from build123d import *

# Parameters (mm, degrees)
SALIENTE_EXTRUIR1_DEPTH     = 180
REDONDEO1_R                 = 100
REDONDEO2_R                 = 10
CROQUIS2_W                  = 140
CROQUIS2_H                  = 70
CORTAR_EXTRUIR4_DEPTH       = 90
CROQUIS3_R                  = 30
CORTAR_EXTRUIR5_DEPTH       = 242.078733734
CORTAR_EXTRUIR6_DEPTH       = 282.806134391
CROQUIS5_W                  = 80.263157895
CROQUIS5_H                  = 10
CORTAR_EXTRUIR8_DEPTH       = 70
CROQUIS6_W                  = 80.263157895
CROQUIS6_H                  = 10
CORTAR_EXTRUIR9_DEPTH       = 243.676183384
REDONDEO8_R                 = 10
CORTAR_EXTRUIR10_DEPTH      = 242.078733734
CORTAR_EXTRUIR10_DEPTH_BACK = 242.078733734
CROQUIS8_W                  = 140
CROQUIS8_H                  = 70
SALIENTE_EXTRUIR2_DEPTH     = 10
CROQUIS9_R                  = 18.735611047
CORTAR_EXTRUIR11_DEPTH      = 282.806134525
REDONDEO9_R                 = 10


# Some blends are built 0.0001 mm under size
with BuildPart() as part:
    # Croquis1 → Saliente-Extruir1 (new body)
    with BuildSketch(Plane.XY):
        Polygon((-15.059146237, -60.657894737), (84.940853763, -60.657894737), (84.940853763, 29.342105263), (4.677695868, 29.342105263), (4.677695868, 139.342105263), (-15.059146237, 139.342105263), align=None)
    extrude(amount=SALIENTE_EXTRUIR1_DEPTH)

    # Redondeo1
    # the kernel refuses this fillet: 100 mm, written as the material it takes off along each edge
    with BuildSketch(Plane(origin=(254.677695868, 139.342105263, 180), x_dir=(0, 0, -1), z_dir=(-1, 0, 0))) as redondeo1_piece_1:
        with BuildLine():
            CenterArc((REDONDEO1_R, REDONDEO1_R), REDONDEO1_R, 180, 90)
            Line((0, REDONDEO1_R), (0, 0))
            Line((0, 0), (REDONDEO1_R, 0))
        make_face()
    extrude(amount=519.736842105, mode=Mode.SUBTRACT)
    with BuildSketch(Plane(origin=(254.677695868, 139.342105263, 0), x_dir=(0, 0, 1), z_dir=(-1, 0, 0))) as redondeo1_piece_2:
        with BuildLine():
            CenterArc((REDONDEO1_R, -REDONDEO1_R), REDONDEO1_R, 90, 90)
            Line((0, -REDONDEO1_R), (0, 0))
            Line((0, 0), (REDONDEO1_R, 0))
        make_face()
    extrude(amount=519.736842105, mode=Mode.SUBTRACT)

    # Redondeo2
    redondeo2_edges = [part.edges().sort_by_distance(p)[0] for p in [
        (44.809274816, 29.342105263, 180),
        (44.809274816, 29.342105263, 0),
    ]]
    fillet(redondeo2_edges, radius=REDONDEO2_R)

    # Croquis2 → Cortar-Extruir4 (cut)
    with BuildSketch(Plane(origin=(84.940853763, 0, 0), x_dir=(0, 0, -1), z_dir=(1, 0, 0))):
        with Locations((-90, -5.657894737)):
            Rectangle(CROQUIS2_W, CROQUIS2_H)
    extrude(amount=-CORTAR_EXTRUIR4_DEPTH, mode=Mode.SUBTRACT)

    # Croquis3 → Cortar-Extruir5 (cut, through all)
    with BuildSketch(Plane(origin=(4.677695868, 0, 0), x_dir=(0, 0, -1), z_dir=(1, 0, 0))):
        with Locations((-90, 93.548562432)):
            Circle(CROQUIS3_R)
    extrude(amount=-CORTAR_EXTRUIR5_DEPTH, mode=Mode.SUBTRACT)

    # Croquis4 → Cortar-Extruir6 (cut, through all)
    with BuildSketch(Plane(origin=(0, -60.657894737, 0), x_dir=(-1, 0, 0), z_dir=(0, -1, 0))):
        with BuildLine():
            Line((-58.010173511, -150), (-58.010173511, -120))
            ThreePointArc((-58.010173511, -120), (-38.975513637, -100.965340126), (-19.940853763, -120))
            Line((-19.940853763, -120), (-19.940853763, -150))
            ThreePointArc((-19.940853763, -150), (-38.975513637, -169.034659874), (-58.010173511, -150))
        make_face()
        with BuildLine():
            Line((-58.010173511, -60), (-58.010173511, -30))
            ThreePointArc((-58.010173511, -30), (-38.975513637, -10.965340126), (-19.940853763, -30))
            Line((-19.940853763, -30), (-19.940853763, -60))
            ThreePointArc((-19.940853763, -60), (-38.975513637, -79.034659874), (-58.010173511, -60))
        make_face()
    extrude(amount=-CORTAR_EXTRUIR6_DEPTH, mode=Mode.SUBTRACT)

    # Croquis5 → Cortar-Extruir8 (cut)
    with BuildSketch(Plane(origin=(0, 29.342105263, 0), x_dir=(1, 0, 0), z_dir=(0, 1, 0))):
        with Locations((44.809274816, -15)):
            Rectangle(CROQUIS5_W, CROQUIS5_H)
        with Locations((44.809274816, -165)):
            Rectangle(CROQUIS5_W, CROQUIS5_H)
    extrude(amount=-CORTAR_EXTRUIR8_DEPTH, mode=Mode.SUBTRACT)

    # Croquis6 → Cortar-Extruir9 (cut, through all)
    with BuildSketch(Plane.XY.offset(180)):
        with Locations((44.809274816, 24.342105263)):
            Rectangle(CROQUIS6_W, CROQUIS6_H)
    extrude(amount=-CORTAR_EXTRUIR9_DEPTH, mode=Mode.SUBTRACT)

    # Redondeo8
    redondeo8_edges = [part.edges().sort_by_distance(p)[0] for p in [
        (84.940853763, 19.342105263, 175),
        (84.940853763, 19.342105263, 5),
    ]]
    fillet(redondeo8_edges, radius=REDONDEO8_R)

    # Croquis7 → Cortar-Extruir10 (cut, two sides: drawn at the far end of the back side and taken through both)
    with BuildSketch(Plane(origin=(4.677695868, 0, 0), x_dir=(0, 0, -1), z_dir=(1, 0, 0)).offset(-CORTAR_EXTRUIR10_DEPTH_BACK)):
        with BuildLine():
            add(Edge.make_bspline(
                [(-113.081277055, 133.711746083), (-124.698414262, 126.957224262), (-152.328432442, 87.000878261), (-154.754506131, 42.525291557), (-180, 19.342105263)],
                knots=[0.150275034, 0.150275034, 0.150275034, 0.150275034, 0.412965146, 1, 1, 1, 1], degree=3))
            ThreePointArc((-113.081277055, 133.711746083), (-161.572445426, 97.186172783), (-180, 39.342105263))
            Line((-180, 39.342105263), (-180, 19.342105263))
        make_face()
        with BuildLine():
            ThreePointArc((0, 39.342105263), (-18.427554574, 97.186172783), (-66.918722945, 133.711746083))
            add(Edge.make_bspline(
                [(-66.918722945, 133.711746083), (-55.301585738, 126.957224262), (-27.671567558, 87.000878261), (-25.245493869, 42.525291557), (0, 19.342105263)],
                knots=[0.150275034, 0.150275034, 0.150275034, 0.150275034, 0.412965146, 1, 1, 1, 1], degree=3))
            Line((0, 19.342105263), (0, 39.342105263))
        make_face()
    extrude(amount=CORTAR_EXTRUIR10_DEPTH + CORTAR_EXTRUIR10_DEPTH_BACK, mode=Mode.SUBTRACT)

    # Croquis8 → Saliente-Extruir2 (add)
    with BuildSketch(Plane(origin=(-5.059146237, 0, 0), x_dir=(0, 0, -1), z_dir=(1, 0, 0))):
        with Locations((-90, -5.657894737)):
            Rectangle(CROQUIS8_W, CROQUIS8_H)
    extrude(amount=SALIENTE_EXTRUIR2_DEPTH)

    # Croquis9 → Cortar-Extruir11 (cut, through all)
    with BuildSketch(Plane.XZ.offset(60.657894737)):
        with Locations((85.924060677, 90)):
            Circle(CROQUIS9_R)
    extrude(amount=-CORTAR_EXTRUIR11_DEPTH, mode=Mode.SUBTRACT)

    # Redondeo9
    redondeo9_edges = [part.edges().sort_by_distance(p)[0] for p in [
        (4.677695868, -10.657894737, 170),
        (4.677695868, -10.657894737, 10),
    ]]
    fillet(redondeo9_edges, radius=REDONDEO9_R - 0.0001)  # a hair under: the kernel refuses the full size


solid = part.part
Build history of the part. All positions in model axes, mm. A direction names the side the tool comes from. Coordinates: 2 decimals unless noted, no trailing zeros. Write each loop counter-clockwise with the first axis right and the second up, starting at its lowest first coordinate (ties: lowest second). Pieces come first, ordered by that corner, then holes.
(1) Pin check, flat tips, straight feed: pin 1 Ø10 at (y, z) = (55.5, 84.5) entering from +X; pin 2 Ø10 at (x, z) = (27.5, 86) entering from +Y; pin 3 Ø22 at (x, z) = (45.5, 165.5) entering from +Y. Stop position of each tip, or through.
(2) Cut at B-B on x = 79. List the corners of the cut face in (y, z).
(3) 3-axis set-ups, long thin cutter, end or side, ignore diameter. For faces 5 (the flat face through (49, -10, 170)), 6 (the cylindrical face through (39.39, -50.8, 10.97)), 7 (the flat face through (34, -20, 0)): which of +Z, -Z, +X, -X, +Y, -Y reach the whole face in a straight line?
(4) Cut at A-A on z = 87. List the corners of the cut face in (x, y).
(5) Mould opens along X. For faces 1 (the cylindrical face through (-5.053, 136.997, 78.469)), 2 (the flat face through (19.941, -51, 135)), 3 (the cylindrical face through (82.089, 16.335, 4.93)), 4 (the flat face through (-15.059, 18, 89)) say: pulls with the +X half, pulls with the -X half, needs draft (parallel to the pull), parting line crosses it, or undercut.
(6) Drill centre lines: line 1 (Z direction, x = 17, y = -20); line 2 (Y direction, x = 14, z = 25.5); line 3 (X direction, y = -39, z = 130.5). Where is each one in solid material? Low to high.
Working result:
1. pin 1: stops at x = 4.68
1. pin 2: stops at y = -40.66
1. pin 3: stops at y = 19.34
2. outline: (-60.66, 0) - (18.48, 0) - (18.48, 10) - (-40.66, 10) - (-40.66, 72.59) - (-60.66, 72.59) - close; (-60.66, 107.41) - (-40.66, 107.41) - (-40.66, 170) - (18.48, 170) - (18.48, 180) - (-60.66, 180) - close
3. face 5: +X, +Y
3. face 6: +Y, -Y
3. face 7: -Z, +X, -X, +Y, -Y
4. outline: (-15.06, -60.66) - (67.43, -60.66) - (67.43, -40.66) - (4.94, -40.66) - (4.94, 29.34) - (4.68, 29.34) - (4.68, 63.7) - (-15.06, 63.7) - close; (-15.06, 123.4) - (4.68, 123.4) - (4.68, 138.49) - (-15.06, 138.49) - close
5. face 1: needs draft
5. face 2: undercut
5. face 3: pulls with the +X half
5. face 4: pulls with the -X half
6. line 1: z = 0 to 10, 170 to 180
6. line 2: y = -60.66 to -40.66
6. line 3: x = -15.06 to 4.94
